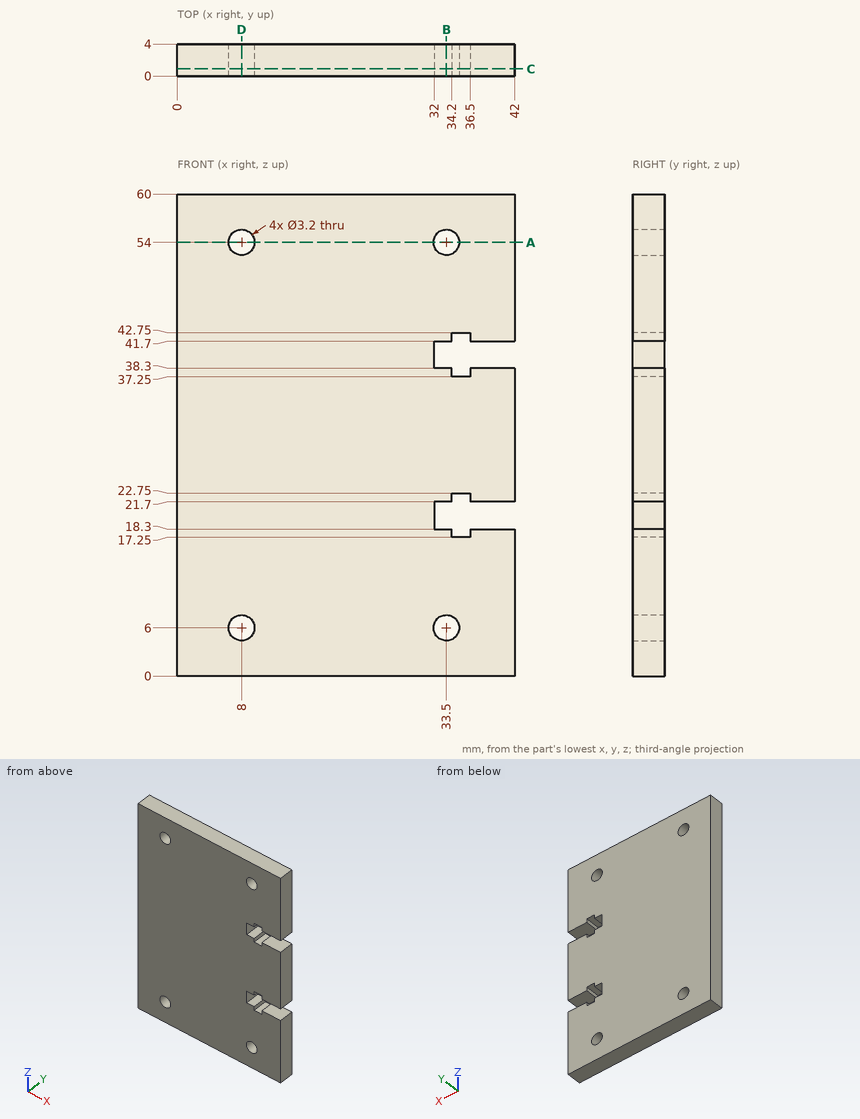
Verification items for this drawing (mm, ordinates from the low corner). Coordinates: 2 decimals unless noted, no trailing zeros. Order: outer loops, then holes, each group sorted by start corner. A loop starts at its lowest first (then second) coordinate and runs counter-clockwise, first axis right, second up. Notation, with made-up numbers: M 58.25,28 L 80.25,28 A19 cw 80.25,64 Z; hole C -3.5,42.5 d5. An arc over 180 degrees is marked long. Write each question's results on one line, items separated by ' | '.
1) Section check A-A on z = 54. Record the cut outline in (x, y), plus the area to 3 significant figures.
Solved:
outline: M 0,0 L 6.4,0 L 6.4,4 L 0,4 Z; M 9.6,0 L 31.9,0 L 31.9,4 L 9.6,4 Z; M 35.1,0 L 42,0 L 42,4 L 35.1,4 Z | area: 142 mm²
2) Scan lines: line 1 along Z through (x, y) = (8, 1.55); line 2 along Z through (x, y) = (35.5, 2.5); line 3 along X through (y, z) = (1, 54). Record each from-to range of solid material in increasing order. Write a range as [from, to].
Solved:
line 1: z = [0, 4.4], [7.6, 52.4], [55.6, 60] | line 2: z = [0, 17.25], [22.75, 37.25], [42.75, 60] | line 3: x = [0, 6.4], [9.6, 31.9], [35.1, 42]
3) Section check B-B on x = 33.5. Record the cut outline in (y, z).
Solved:
outline: M 0,0 L 4,0 L 4,4.4 L 0,4.4 Z; M 0,7.6 L 4,7.6 L 4,18.3 L 0,18.3 Z; M 0,21.7 L 4,21.7 L 4,38.3 L 0,38.3 Z; M 0,41.7 L 4,41.7 L 4,52.4 L 0,52.4 Z; M 0,55.6 L 4,55.6 L 4,60 L 0,60 Z
4) Section check C-C on y = 0.9. Give the number of separate pieces and of enclosed holes in the cut face, plus the area to 3 significant figures.
Solved:
separate pieces: 1 | enclosed holes: 4 | area: 2,410 mm²
5) Section check D-D on x = 8. Record the cut outline in (y, z), plus the area to 3 significant figures.
Solved:
outline: M 0,0 L 4,0 L 4,4.4 L 0,4.4 Z; M 0,7.6 L 4,7.6 L 4,52.4 L 0,52.4 Z; M 0,55.6 L 4,55.6 L 4,60 L 0,60 Z | area: 214 mm²
6) Gauge pin test, flat ends, axial feed: pin 1 Ø2 at (y, z) = (2.5, 24) entering from -X; pin 2 Ø1 at (y, z) = (3, 40.5) entering from +X. Record the tip position at first contact, or that the pin passes through.
Solved:
pin 1: stops at x = 0 | pin 2: stops at x = 32
